Source: CAD feature listing. Evaluate the final solid. Frame: model axes, mm. A direction names the side the tool comes from. Coordinates: 2 decimals unless noted, no trailing zeros. Write each loop counter-clockwise with the first axis right and the second up, starting at its lowest first coordinate (ties: lowest second). Pieces come first, ordered by that corner, then holes. Notation, with made-up numbers: M 53.5,-32 L 103.5,-32 A29 ccw 103.5,-7 Z; hole C 4.5,-1.75 d10. An arc over 180 degrees is marked long. One line per item, written item: value. Start each with the question number.
Item 1: Mould query, pull axis X, two halves, no side actions, for faces 4 (the cylindrical face through (1.341, -3.233, 10.024)), 5 (the conical face through (0.82, -1.39, 11.88)), 6 (the flat face through (1, 2, 8)). Classes: released by +X, released by -X, zero draft, split by the parting line, or undercut.
Item 2: Cut plane A-A, the plane z = -8.5. Output: boundary loops of the cut face in (x, y).
Item 3: Set-up query: faces 1 (the conical face through (-0.8, -1.4, 11.88)), 2 (the flat face through (0, 0, -12)), 3 (the cylindrical face through (2, 0, -2)). Return all of +Z, -Z, +X, -X, +Y, -Y with unobstructed straight access to the full face (end or side cutting, diameter ignored); none if empty.
Item 4: Ray query, L1, parallel to Z at x = 1.5, y = 1.5; L2, parallel to X at y = -1, z = 1.75; L3, parallel to X at y = 0, z = 9.75. Return the intervals inside material, ascending. Write a range as from..to.
Item 5: Pin query (flat end, axial travel): P1, Ø1.5, axis at y = 2.5, z = -3.5, coming from the -X side; P2, Ø3, axis at x = 2, z = 0, coming from the -Y side; P3, Ø1, axis at y = -1.5, z = 5.5, coming from the -X side. Return the tip coordinate at first contact, or that it passes through.
```python
from build123d import *

# Parameters (mm, degrees)
CUT_EXTRUDE1_DEPTH = 2


with BuildPart() as part:
    # Sketch3 → Revolve1 (revolve)
    with BuildSketch(Plane(origin=(0, 0, 0), x_dir=(0, 0, -1), z_dir=(1, 0, 0)), mode=Mode.PRIVATE) as revolve1_sk:
        with BuildLine():
            Line((-12, 3.191005051), (-12, 1.5))
            Line((-12, 1.5), (-10, 1.5))
            Line((-10, 1.5), (-10, 0))
            Line((-10, 0), (12, 0))
            Line((12, 0), (12, 1.545336663))
            Line((12, 1.545336663), (11.545336663, 2))
            Line((11.545336663, 2), (-8, 2))
            Line((-8, 2), (-8, 3.191005051))
            ThreePointArc((-8, 3.191005051), (-8.005328433, 3.217792891), (-8.020502525, 3.240502525))
            Line((-8.020502525, 3.240502525), (-8.259497475, 3.479497475))
            ThreePointArc((-8.259497475, 3.479497475), (-8.282207109, 3.494671567), (-8.308994949, 3.5))
            Line((-8.308994949, 3.5), (-11.691005051, 3.5))
            ThreePointArc((-11.691005051, 3.5), (-11.717792891, 3.494671567), (-11.740502525, 3.479497475))
            Line((-11.740502525, 3.479497475), (-11.979497475, 3.240502525))
            ThreePointArc((-11.979497475, 3.240502525), (-11.994671567, 3.217792891), (-12, 3.191005051))
        make_face()
    revolve(revolve1_sk.sketch.rotate(Axis((0, 0, 12), (0, 0, -1)), 180), axis=Axis((0, 0, 12), (0, 0, -1)))

    # Sketch4 → Cut-Extrude1 (cut)
    with BuildSketch(Plane.XY.offset(12)):
        Polygon((0, 1.732050808), (-1.5, 0.866025404), (-1.5, -0.866025404), (0, -1.732050808), (1.5, -0.866025404), (1.5, 0.866025404), align=None)
    extrude(amount=-CUT_EXTRUDE1_DEPTH, mode=Mode.SUBTRACT)

    # Cut-Extrude2 cone 1 section (through the dimple's axis) → Cut-Extrude2 (revolve, cut)
    with BuildSketch(Plane(origin=(0, 0, 12), x_dir=(0, -1, 0), z_dir=(1, 0, 0))):
        Polygon((0, 0), (1.732050808, 0), (0, 1.732050808), align=None)
    revolve(axis=Axis((0, 0, 12), (0, 0, -1)), mode=Mode.SUBTRACT)

    # Cut-Extrude3 cone 1 section (through the dimple's axis) → Cut-Extrude3 (revolve, cut)
    with BuildSketch(Plane(origin=(0, 0, 10), x_dir=(0, -1, 0), z_dir=(1, 0, 0))):
        Polygon((0, 0), (1.5, 0), (0, 0.866025404), align=None)
    revolve(axis=Axis((0, 0, 10), (0, 0, -1)), mode=Mode.SUBTRACT)


solid = part.part
```
From the geometry:
1. face 4: split by the parting line
1. face 5: undercut
1. face 6: zero draft
2. outline: C 0,0 d4
3. face 1: +Z
3. face 2: -Z, +X, -X, +Y, -Y
3. face 3: -Z
4. L1: z = 8..12
4. L2: x = -1.73..1.73
4. L3: x = -3.5..-1.07, 1.07..3.5
5. P1: stops at x = -0.97
5. P2: stops at y = -1.94
5. P3: stops at x = -1.73
